Input: part model. Units: mm. Frame: model coordinates. Face numbers are marked on the shaded views. A direction names the side the tool comes from. Coordinates: 2 decimals unless noted, no trailing zeros. Write each loop counter-clockwise with the first axis right and the second up, starting at its lowest first coordinate (ties: lowest second). Pieces come first, ordered by that corner, then holes. Notation, with made-up numbers: M 41.25,58 L 87.25,58 A20 ccw 87.25,78 Z; hole C 34.25,7 d2. An arc over 180 degrees is marked long. Use CSV: the item, a comma, the result in double quotes.
```python
from build123d import *

# Parameters (mm, degrees)
SKETCH2_R          = 1.5
CUT_EXTRUDE1_DEPTH = 32.769836323


with BuildPart() as part:
    # Sketch1 → Revolve1 (revolve)
    with BuildSketch(Plane.XY, mode=Mode.PRIVATE) as revolve1_sk:
        Polygon((-13.325, 1), (-13.325, 15), (-10.325, 15), (-10.325, 5), (-5.975, 5), (-5.975, 4), (3.325, 4), (3.325, 2), (13.325, 2), (13.325, 1), align=None)
    revolve(revolve1_sk.sketch.rotate(Axis((-13.325, 0, 0), (1, 0, 0)), 90), axis=Axis((-13.325, 0, 0), (1, 0, 0)))

    # Sketch2 → Cut-Extrude1 (cut, through all)
    with BuildSketch(Plane(origin=(-10.325, 0, 0), x_dir=(0, 0, -1), z_dir=(1, 0, 0))):
        with Locations((0, 10)):
            Circle(SKETCH2_R)
        with Locations((10, 0)):
            Circle(SKETCH2_R)
        with Locations((0, -10)):
            Circle(SKETCH2_R)
        with Locations((-10, 0)):
            Circle(SKETCH2_R)
    extrude(amount=-CUT_EXTRUDE1_DEPTH, mode=Mode.SUBTRACT)


solid = part.part
```
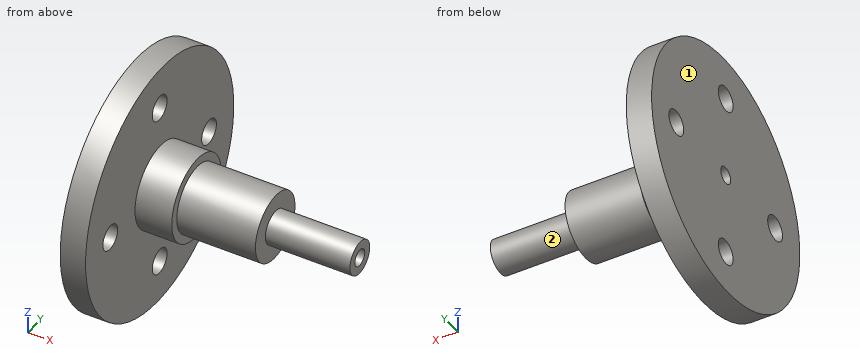
1. Access query for the marked faces 1 and 2. Directions: +Z, -Z, +X, -X, +Y, -Y. A direction counts if a zero-diameter tool reaches every point of the face in a straight line with its end or side. Return the directions, or none.
Resolved:
face 1,"+Z, -Z, -X, +Y, -Y"
face 2,"+X"
2. Section B-B (z = 10). Return loops of the section in (x, y) (3 decimals), then the cut area to 3 significant figures.
Resolved:
outline,"M -13.325,-11.18 L -10.325,-11.18 L -10.325,-1.5 L -13.325,-1.5 Z; M -13.325,1.5 L -10.325,1.5 L -10.325,11.18 L -13.325,11.18 Z"
area,"58.1 mm^2"
3. Material intervals for line 1 (Y direction, x = -11.25, z = 0); line 2 (Y direction, x = -7, z = 0); line 3 (X direction, y = 8.5, z = -11.25) (3 decimals), sorted ascending. Write a range as [from, to].
Resolved:
line 1,"y = [-15, -11.5], [-8.5, -1], [1, 8.5], [11.5, 15]"
line 2,"y = [-5, -1], [1, 5]"
line 3,"x = [-13.325, -10.325]"
4. Contact query for flat-ended pins moving along their axis: pin 1 Ø1.8 at (y, z) = (0, 10) entering from -X; pin 2 Ø2 at (x, z) = (-9.5, 5) entering from +Y; pin 3 Ø3 at (y, z) = (-11, -11.5) entering from -X (3 decimals); pin 4 Ø6 at (y, z) = (5.5, 5.5) entering from +X (3 decimals). Output: stop coordinate, or through.
Resolved:
pin 1,"passes through"
pin 2,"stops at y = 14.33"
pin 3,"stops at x = -13.325"
pin 4,"stops at x = -5.975"
5. Section A-A (z = 0). Return loops of the section in (x, y) (3 decimals).
Resolved:
outline,"M -13.325,-15 L -10.325,-15 L -10.325,-11.5 L -13.325,-11.5 Z; M -13.325,-8.5 L -10.325,-8.5 L -10.325,-5 L -5.975,-5 L -5.975,-4 L 3.325,-4 L 3.325,-2 L 13.325,-2 L 13.325,-1 L -13.325,-1 Z; M -13.325,1 L 13.325,1 L 13.325,2 L 3.325,2 L 3.325,4 L -5.975,4 L -5.975,5 L -10.325,5 L -10.325,8.5 L -13.325,8.5 Z; M -13.325,11.5 L -10.325,11.5 L -10.325,15 L -13.325,15 Z"
6. Section D-D (x = 1). Return loops of the section in (y, z).
Resolved:
outline,"C 0,0 d8; hole C 0,0 d2"
